Build history of the part. All positions in model axes, mm. A direction names the side the tool comes from. Round coordinates to 2 decimals unless told otherwise and drop trailing zeros. Loops run counter-clockwise (first coordinate to the right, second up) from the corner with the lowest first, then second, coordinate; pieces in that order, holes last. Notation, with made-up numbers: (5.5, 7.5) - (64.5, 7.5) arc R19 ccw to (64.5, 31.5) - close; hole circle Ø5 at (43.5, -37). An arc over 180 degrees is marked (long way). Use one line per item in the form item = value. Start each with the question number.
Q1. 3-axis set-ups, long thin cutter, end or side, ignore diameter. For faces 4 (the face through (5, -16.171, 8)), 5 (the face through (-16.517, -21.101, -22.191)), 6 (the face through (-31.374, 73, 18)), 7 (the face through (-31.374, 73, -18)): which of +Z, -Z, +X, -X, +Y, -Y reach the whole face in a straight line?
Q2. Drill centre lines: line 1 (X direction, y = 63, z = -28.5); line 2 (Z direction, x = -29, y = 126.5); line 3 (Y direction, x = -11, z = 27.5). Where is each one in solid material? Low to high.
Q3. Saw through at B-B (x = -5.5). Give the cut face in (y, z), then the cut area to 3 significant figures.
Q4. Saw through at C-C (y = 66). Give the cut face in (x, z), then the cut area to 3 significant figures.
Q5. Pin check, flat tips, straight feed: pin 1 (4.5 mm diameter, centred on x = 20.63, z = -20, fed in from -Y); pin 2 (1 mm diameter, centred on y = 135.5, z = -5, fed in from -X); pin 3 (6 mm diameter, centred on x = -27, y = 82.5, fed in from +Z); pin 4 (9.5 mm diameter, centred on x = -19.37, z = -20, fed in from -Y). Stop position of each tip, or through.
Q6. Saw through at A-A (z = 20). Give the cut face in (x, y).
Q7. Saw through at D-D (z = -20). Give the cut face in (x, y).
Q8. Mould opens along Z. For faces 1 (the face through (36.12, -21.1, 28.22)), 2 (the face through (-19, 35, -4)), 3 (the face through (-16.517, -21.101, 17.809)) say: released by +Z, released by -Z, zero draft, split by the parting line, or undercut.
```python
from build123d import *

# Parameters (mm, degrees)
AUFSATZ_LINEAR_AUSTRAGEN1_DEPTH = 32.5
AUFSATZ_LINEAR_AUSTRAGEN2_DEPTH = 4
SKIZZE4_W                       = 26
SKIZZE4_H                       = 42
SCHNITT_LINEAR_AUSTRAGEN1_DEPTH = 2
SKIZZE5_R                       = 1.4
SCHNITT_LINEAR_AUSTRAGEN2_DEPTH = 10
SKIZZE6_W                       = 34.028268395
SKIZZE6_H                       = 30
SCHNITT_LINEAR_AUSTRAGEN3_DEPTH = 2
SKIZZE7_R                       = 3.6
SCHNITT_LINEAR_AUSTRAGEN4_DEPTH = 10
VERRUNDUNG1_R                   = 15


with BuildPart() as part:
    # Skizze1 → Aufsatz-Linear austragen1 (new, symmetric)
    with BuildSketch(Plane.XY):
        Polygon((-39.374028295, 163.828996283), (-39.374028295, -26.171003717), (40.625971705, -26.171003717), (40.625971705, -16.171003717), (-31.374028295, -16.171003717), (-31.374028295, 163.828996283), align=None)
    extrude(amount=AUFSATZ_LINEAR_AUSTRAGEN1_DEPTH, both=True)

    # Skizze2 → Aufsatz-Linear austragen2 (add, symmetric)
    with BuildSketch(Plane.XY):
        Polygon((-31.374028295, 163.828996283), (13.784951867, -16.171003717), (-31.374028295, -16.171003717), align=None)
    extrude(amount=AUFSATZ_LINEAR_AUSTRAGEN2_DEPTH, both=True)

    # Skizze4 → Schnitt-Linear austragen1 (cut)
    with BuildSketch(Plane.ZY.offset(39.374028295)):
        with Locations((0, 142.828996283)):
            Rectangle(SKIZZE4_W, SKIZZE4_H)
    extrude(amount=-SCHNITT_LINEAR_AUSTRAGEN1_DEPTH, mode=Mode.SUBTRACT)

    # Skizze5 → Schnitt-Linear austragen2 (cut)
    with BuildSketch(Plane.ZY.offset(37.374028295)):
        with Locations(Location((-9.5, 124.828996283, 0), (0, 0, 270))):
            Circle(SKIZZE5_R)
        with Locations(Location((9.5, 124.828996283, 0), (0, 0, 270))):
            Circle(SKIZZE5_R)
        with Locations(Location((-9.5, 131.158996283, 0), (0, 0, 270))):
            Circle(SKIZZE5_R)
        with Locations(Location((9.5, 131.158996283, 0), (0, 0, 270))):
            Circle(SKIZZE5_R)
        with Locations(Location((-9.5, 137.488996283, 0), (0, 0, 270))):
            Circle(SKIZZE5_R)
        with Locations(Location((9.5, 137.488996283, 0), (0, 0, 270))):
            Circle(SKIZZE5_R)
        with Locations(Location((-9.5, 143.818996283, 0), (0, 0, 270))):
            Circle(SKIZZE5_R)
        with Locations(Location((9.5, 143.818996283, 0), (0, 0, 270))):
            Circle(SKIZZE5_R)
        with Locations(Location((-9.5, 150.148996283, 0), (0, 0, 270))):
            Circle(SKIZZE5_R)
        with Locations(Location((9.5, 150.148996283, 0), (0, 0, 270))):
            Circle(SKIZZE5_R)
        with Locations(Location((-9.5, 156.478996283, 0), (0, 0, 270))):
            Circle(SKIZZE5_R)
        with Locations(Location((9.5, 156.478996283, 0), (0, 0, 270))):
            Circle(SKIZZE5_R)
    extrude(amount=-SCHNITT_LINEAR_AUSTRAGEN2_DEPTH, mode=Mode.SUBTRACT)

    # Skizze6 → Schnitt-Linear austragen3 (cut)
    with BuildSketch(Plane.ZY.offset(39.374028295)):
        with Locations((17.014134198, 149.158996283)):
            Rectangle(SKIZZE6_W, SKIZZE6_H)
    extrude(amount=-SCHNITT_LINEAR_AUSTRAGEN3_DEPTH, mode=Mode.SUBTRACT)

    # Skizze7 → Schnitt-Linear austragen4 (cut)
    with BuildSketch(Plane(origin=(0, -16.171003717, 0), x_dir=(1, 0, 0), z_dir=(0, 1, 0))):
        with Locations(Location((20.625971705, 20, 0), (0, 0, 180))):
            Circle(SKIZZE7_R)
        with Locations(Location((20.625971705, -20, 0), (0, 0, 180))):
            Circle(SKIZZE7_R)
        with Locations(Location((-19.374028295, 20, 0), (0, 0, 180))):
            Circle(SKIZZE7_R)
        with Locations(Location((-19.374028295, -20, 0), (0, 0, 180))):
            Circle(SKIZZE7_R)
    extrude(amount=-SCHNITT_LINEAR_AUSTRAGEN4_DEPTH, mode=Mode.SUBTRACT)

    # Verrundung1
    verrundung1_edges = [part.edges().sort_by_distance(p)[0] for p in [
        (40.625971705, -21.171003717, 32.5),
        (40.625971705, -21.171003717, -32.5),
    ]]
    fillet(verrundung1_edges, radius=VERRUNDUNG1_R)


solid = part.part
```
Report:
q1.face_4 = +X, +Y
q1.face_5 = +Y, -Y
q1.face_6 = +Z, +X, +Y
q1.face_7 = -Z, +X, +Y
q2.line_1 = -39.37 to -31.37
q2.line_2 = -4 to 4
q2.line_3 = -26.17 to -16.17
q3.outline = (-26.17, -32.5) - (-16.17, -32.5) - (-16.17, -4) - (60.7, -4) - (60.7, 4) - (-16.17, 4) - (-16.17, 32.5) - (-26.17, 32.5) - close
q3.area = 1,260 mm²
q4.outline = (-39.37, -32.5) - (-31.37, -32.5) - (-31.37, -4) - (-6.83, -4) - (-6.83, 4) - (-31.37, 4) - (-31.37, 32.5) - (-39.37, 32.5) - close
q4.area = 716 mm²
q5.pin_1 = through
q5.pin_2 = -37.37
q5.pin_3 = 4
q5.pin_4 = -26.17
q6.outline = (-39.37, -26.17) - (-22.97, -26.17) - (-22.97, -16.17) - (-31.37, -16.17) - (-31.37, 163.83) - (-37.37, 163.83) - (-37.37, 134.16) - (-39.37, 134.16) - close; (-15.77, -26.17) - (17.03, -26.17) - (17.03, -16.17) - (-15.77, -16.17) - close; (24.23, -26.17) - (40.42, -26.17) - (40.42, -16.17) - (24.23, -16.17) - close
q7.outline = (-39.37, -26.17) - (-22.97, -26.17) - (-22.97, -16.17) - (-31.37, -16.17) - (-31.37, 163.83) - (-39.37, 163.83) - close; (-15.77, -26.17) - (17.03, -26.17) - (17.03, -16.17) - (-15.77, -16.17) - close; (24.23, -26.17) - (40.42, -26.17) - (40.42, -16.17) - (24.23, -16.17) - close
q8.face_1 = released by +Z
q8.face_2 = released by -Z
q8.face_3 = undercut
